```python
from build123d import *

# Parameters (mm, degrees)
MX_START           = 53
MX_POD_DEPTH       = 14
MX_START_2         = 65.5
MX_CUTOUT_DEPTH    = 1.7
MX_START_3         = 55
MX_RELIEF_DEPTH    = 10.5
MX_START_4         = 52.8
SKETCH5_R          = 3.5
MX_LEAD_HOLE_DEPTH = 2.4
BOLT_START         = 52.8
SKETCH6_R          = 1.7
BOLT_HOLES_DEPTH   = 6.4


with BuildPart() as part:
    # Sketch1 → Lip ring (revolve)
    with BuildSketch(Plane.XY, mode=Mode.PRIVATE) as lip_ring_sk:
        Polygon((70.5, 53), (82, 53), (82, 59), (66.45, 59), (70.5, 54.95), align=None)
    revolve(lip_ring_sk.sketch.rotate(Axis((0, 40, 0), (0, 1, 0)), 90), axis=Axis((0, 40, 0), (0, 1, 0)))

    # Sketch2 → MX pod (add)
    with BuildSketch(Plane(origin=(0, 0, 0), x_dir=(1, 0, 0), z_dir=(0, 1, 0)).offset(MX_START)):
        with BuildLine():
            Line((-8, 92), (8, 92))
            ThreePointArc((8, 92), (10.828427125, 90.828427125), (12, 88))
            Line((12, 88), (12, 75))
            ThreePointArc((12, 75), (10.828427125, 72.171572875), (8, 71))
            Line((8, 71), (-8, 71))
            ThreePointArc((-8, 71), (-10.828427125, 72.171572875), (-12, 75))
            Line((-12, 75), (-12, 88))
            ThreePointArc((-12, 88), (-10.828427125, 90.828427125), (-8, 92))
        make_face()
    extrude(amount=MX_POD_DEPTH)

    # Sketch3 → MX cutout (cut)
    with BuildSketch(Plane(origin=(0, 0, 0), x_dir=(1, 0, 0), z_dir=(0, 1, 0)).offset(MX_START_2)):
        with BuildLine():
            Line((-6.65, 88.55), (6.65, 88.55))
            ThreePointArc((6.65, 88.55), (6.932842712, 88.432842712), (7.05, 88.15))
            Line((7.05, 88.15), (7.05, 74.85))
            ThreePointArc((7.05, 74.85), (6.932842712, 74.567157288), (6.65, 74.45))
            Line((6.65, 74.45), (-6.65, 74.45))
            ThreePointArc((-6.65, 74.45), (-6.932842712, 74.567157288), (-7.05, 74.85))
            Line((-7.05, 74.85), (-7.05, 88.15))
            ThreePointArc((-7.05, 88.15), (-6.932842712, 88.432842712), (-6.65, 88.55))
        make_face()
    extrude(amount=MX_CUTOUT_DEPTH, mode=Mode.SUBTRACT)

    # Sketch4 → MX relief (cut)
    with BuildSketch(Plane(origin=(0, 0, 0), x_dir=(1, 0, 0), z_dir=(0, 1, 0)).offset(MX_START_3)):
        with BuildLine():
            Line((-7.5, 89.5), (7.5, 89.5))
            ThreePointArc((7.5, 89.5), (7.853553391, 89.353553391), (8, 89))
            Line((8, 89), (8, 74))
            ThreePointArc((8, 74), (7.853553391, 73.646446609), (7.5, 73.5))
            Line((7.5, 73.5), (-7.5, 73.5))
            ThreePointArc((-7.5, 73.5), (-7.853553391, 73.646446609), (-8, 74))
            Line((-8, 74), (-8, 89))
            ThreePointArc((-8, 89), (-7.853553391, 89.353553391), (-7.5, 89.5))
        make_face()
    extrude(amount=MX_RELIEF_DEPTH, mode=Mode.SUBTRACT)

    # Sketch5 → MX lead hole (cut)
    with BuildSketch(Plane(origin=(0, 0, 0), x_dir=(1, 0, 0), z_dir=(0, 1, 0)).offset(MX_START_4)):
        with Locations(Location((0, 76.5, 0), (0, 0, 90))):
            Circle(SKETCH5_R)
    extrude(amount=MX_LEAD_HOLE_DEPTH, mode=Mode.SUBTRACT)

    # Sketch6 → Bolt holes (cut)
    with BuildSketch(Plane(origin=(0, 0, 0), x_dir=(1, 0, 0), z_dir=(0, 1, 0)).offset(BOLT_START)):
        with Locations(Location((76.5, 0, 0), (0, 0, 90))):
            Circle(SKETCH6_R)
        with Locations(Location((38.25, -66.25094339, 0), (0, 0, 90))):
            Circle(SKETCH6_R)
        with Locations(Location((-38.25, -66.25094339, 0), (0, 0, 90))):
            Circle(SKETCH6_R)
        with Locations(Location((-76.5, 0, 0), (0, 0, 90))):
            Circle(SKETCH6_R)
        with Locations(Location((-38.25, 66.25094339, 0), (0, 0, 90))):
            Circle(SKETCH6_R)
        with Locations(Location((38.25, 66.25094339, 0), (0, 0, 90))):
            Circle(SKETCH6_R)
    extrude(amount=BOLT_HOLES_DEPTH, mode=Mode.SUBTRACT)


solid = part.part
```
The listing builds one solid part. Answer for the finished solid, in the listing's coordinates (mm). A direction names the side the tool comes from. Give positions to 0.01 mm unless a question says otherwise; leave off trailing zeros. Loops run counter-clockwise (first coordinate to the right, second up) from the corner with the lowest first, then second, coordinate; pieces in that order, holes last. Notation, with made-up numbers: (43.5, 69) - (96.5, 69) arc R13 ccw to (96.5, 73) - close; hole circle Ø8 at (-34.75, -23). An arc over 180 degrees is marked (long way). Return JSON: item names as keys, results as strings. Group by question number.
1. Find section A-A (y = 63.5). Write down the section's boundary in (x, z).
2. Straight lines are drawn through the part: line 1 (X direction, y = 53.85, z = 0); line 2 (X direction, y = 56, z = -84); line 3 (Y direction, x = 7.5, z = -82). For each, find the intervals that lie inside material, in ascending order. Write a range as [from, to].
3. Determine the mould class of faces 1 (the flat face through (-12, 61, -83)), 2 (the conical face through (65.117, 58.747, 14.46)), 3 (the flat face through (0, 60, -92)), 4 (the flat face through (-8, 60, -81)) for opening direction X: pulls with the +X half, pulls with the -X half, needs draft (parallel to the pull), parting line crosses it, or undercut.
4. Given pin 1 Ø8 at (x, y) = (11, 58.5) entering from +Z; pin 2 Ø5 at (x, z) = (2, -83) entering from +Y; pin 3 Ø0.8 at (y, z) = (66, -83) entering from +X, each flat-ended and moving along its own axis, determine where each tip first touches the part or whether it passes through.
5. Which of the six approach directions +Z, -Z, +X, -X, +Y, -Y give full straight-line access (tool end or side, diameter ignored) to faces 5 (the cylindrical face through (0, 54, -73)), 6 (the cylindrical face through (-10.797, 62.944, -72.141)), 7 (the flat face through (0, 63, -71)), 8 (the flat face through (0, 55, -82)), 9 (the cylindrical face through (10.859, 62.944, -72.203))?
Verdict:
{
 "1": {"outline": "(-12, -88) arc R4 ccw to (-8, -92) - (8, -92) arc R4 ccw to (12, -88) - (12, -75) arc R4 ccw to (8, -71) - (-8, -71) arc R4 ccw to (-12, -75) - close; hole (-8, -89) arc R0.5 ccw to (-7.5, -89.5) - (7.5, -89.5) arc R0.5 ccw to (8, -89) - (8, -74) arc R0.5 ccw to (7.5, -73.5) - (-7.5, -73.5) arc R0.5 ccw to (-8, -74) - close"},
 "2": {"line 1": "x = [-82, -78.2], [-74.8, -70.5], [70.5, 74.8], [78.2, 82]", "line 2": "x = [-12, -8], [8, 12]", "line 3": "y = [53, 55], [65.5, 67]"},
 "3": {"face 1": "pulls with the -X half", "face 2": "undercut", "face 3": "needs draft", "face 4": "undercut"},
 "4": {"pin 1": "stops at z = 81.7", "pin 2": "stops at y = 55", "pin 3": "stops at x = 12"},
 "5": {"face 5": "-Y", "face 6": "+Z, -X, +Y", "face 7": "+Z, +X, -X, +Y", "face 8": "none", "face 9": "+Z, +X, +Y"}
}
